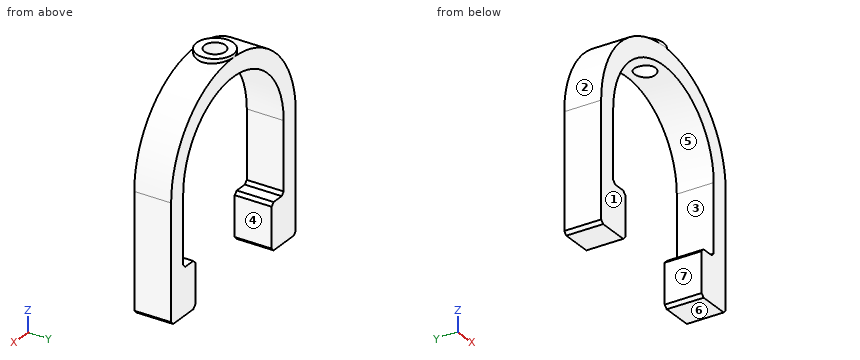
```python
from build123d import *

# Parameters (mm, degrees)
F1_DEPTH = 6
F2_SIZE2 = 1
F2_SIZE  = 1
F4_R     = 6
F5_DEPTH = 1.5861874485
F6_D     = 6.8


with BuildPart() as f1:
    # F0 (on Front) → F1 (new body, symmetric)
    with BuildSketch(Plane.XZ):
        with BuildLine():
            ThreePointArc((-25, 0), (0, 25), (25, 0))
            Line((25, 0), (25, -23))
            Line((25, -23), (19, -23))
            Line((19, -23), (19, -38))
            Line((19, -38), (31, -38))
            Line((31, -38), (31, 0))
            ThreePointArc((31, 0), (0, 31), (-31, 0))
            Line((-31, 0), (-31, -38))
            Line((-31, -38), (-19, -38))
            Line((-19, -38), (-19, -23))
            Line((-19, -23), (-25, -23))
            Line((-25, -23), (-25, 0))
        make_face()
    extrude(amount=F1_DEPTH, both=True)

    # F2
    f2_edges = [f1.edges().sort_by_distance(p)[0] for p in [
        (-25, 0, -23),
        (-19, 0, -23),
        (-19, 0, -38),
        (-31, 0, -38),
        (19, 0, -38),
        (31, 0, -38),
        (25, 0, -23),
        (19, 0, -23),
    ]]
    chamfer(f2_edges, length=F2_SIZE, length2=F2_SIZE2)

    # F4 (on offset) → F5 (join, through all)
    with BuildSketch(Plane.XY.offset(32)):
        Circle(F4_R)
    extrude(amount=-F5_DEPTH)

    # F6 (through all)
    with Locations(Plane.XY.offset(32)):
        with Locations((0, 0)):
            Hole(F6_D / 2)


solid = f1.part
```
For this review, take the finished solid that the model builds, in its own axes (mm). Face numbers are marked on the shaded views. A direction names the side the tool comes from. Round coordinates to 2 decimals unless told otherwise and drop trailing zeros. Loops run counter-clockwise (first coordinate to the right, second up) from the corner with the lowest first, then second, coordinate; pieces in that order, holes last.
(1) We need section C-C (z = -11). Give the boundary of the cut face in (x, y).
Returned:
outline: (-31, -6) - (-25, -6) - (-25, 6) - (-31, 6) - close; (25, -6) - (31, -6) - (31, 6) - (25, 6) - close
(2) We need section B-B (y = 0). Give the boundary of the cut face in (x, z), plus the area to 3 significant figures.
Returned:
outline: (-31, -37) - (-30, -38) - (-20, -38) - (-19, -37) - (-19, -24) - (-20, -23) - (-24, -23) - (-25, -22) - (-25, 0) arc R25 cw to (-3.4, 24.77) - (-3.4, 32) - (-6, 32) - (-6, 30.41) arc R31 ccw to (-31, 0) - close; (3.4, 24.77) arc R25 cw to (25, 0) - (25, -22) - (24, -23) - (20, -23) - (19, -24) - (19, -37) - (20, -38) - (30, -38) - (31, -37) - (31, 0) arc R31 ccw to (6, 30.41) - (6, 32) - (3.4, 32) - close
area: 1,130 mm2
(3) Tool access review of the marked faces 5, 6 and 7: name each direction out of +Z, -Z, +X, -X, +Y, -Y from which nothing blocks a thin tool from reaching the whole face with its end or side.
Returned:
face 5: +Y, -Y
face 6: -Z, +X, -X, +Y, -Y
face 7: -Z, +Y, -Y
(4) Mouldability with a two-part tool opening along X and no side actions: class the marked faces 1, 2, 3 and 4 as released by +X, released by -X, zero draft, split by the parting line, or undercut.
Returned:
face 1: zero draft
face 2: released by -X
face 3: undercut
face 4: undercut
(5) We need section A-A (z = -28). Give the boundary of the cut face in (x, y), plus the area to 3 significant figures.
Returned:
outline: (-31, -6) - (-19, -6) - (-19, 6) - (-31, 6) - close; (19, -6) - (31, -6) - (31, 6) - (19, 6) - close
area: 288 mm2
(6) We need section D-D (y = -4.5). Give the boundary of the cut face in (x, z).
Returned:
outline: (-31, -37) - (-30, -38) - (-20, -38) - (-19, -37) - (-19, -24) - (-20, -23) - (-24, -23) - (-25, -22) - (-25, 0) arc R25 cw to (25, 0) - (25, -22) - (24, -23) - (20, -23) - (19, -24) - (19, -37) - (20, -38) - (30, -38) - (31, -37) - (31, 0) arc R31 ccw to (3.97, 30.74) - (3.97, 32) - (-3.97, 32) - (-3.97, 30.74) arc R31 ccw to (-31, 0) - close
(7) Clearance check with flat-ended pins moving along their axes: P1, Ø1, axis at y = 3, z = 14, coming from the -X side; P2, Ø4, axis at y = -3, z = 6.5, coming from the -X side; P3, Ø1.5, axis at x = -13, y = -2.5, coming from the +Z side. State where each tip first meets the part, or that it passes through.
Returned:
P1: stops at x = -27.91
P2: stops at x = -30.67
P3: stops at z = 28.48
(8) Wall thickness on line 1 along X through (y, z) = (1.5, -11); line 2 along Y through (x, z) = (0, 28.5); line 3 along X through (y, z) = (0, 27): over which ranges is each line inside the solid? List them lowest first.
Returned:
line 1: x = -31 to -25, 25 to 31
line 2: y = -6 to -3.4, 3.4 to 6
line 3: x = -15.23 to -3.4, 3.4 to 15.23
